Autodesk Inventor part; units mm, degrees
ref_plane "YZ Plane" through (0, 0, 0) normal (1, 0, 0) x (0, 1, 0)
ref_plane "XZ Plane" through (0, 0, 0) normal (0, 1, 0) x (-1, 0, 0)
ref_plane "XY Plane" through (0, 0, 0) normal (0, 0, 1) x (1, 0, 0)
sketch "Sketch1" plane through (0, 0, 0) normal (0, 0, 1) x (1, 0, 0)
  line L0 (0, 65.5357) -> (0, 44) construction
  line L1 (0, 0) -> (50, 0)
  line L2 (50, 0) -> (50, 5)
  line L3 (50, 5) -> (25, 5)
  line L4 (25, 5) -> (25, 68)
  line L5 (25, 68) -> (14, 68)
  line L6 (14, 68) -> (14, 58)
  arc A0 (0, 44) -> (14, 58) centre (0, 58) ccw
  circle A1 centre (17.75, 58) radius 2
  line L7 (0, 44) -> (0, 0)
  point P0 (0, 50)
  dimension "d0" = 5
  dimension "d1" = 50
  dimension "d2" = 25
  dimension "d4" = 14
  dimension "d5" = 4
  dimension "d6" = 17.75
  dimension "d7" = 10
  dimension "d22" = 50
  dimension "d23" = 6
extrude "Extrusion1" add sketch "Sketch1" along normal blind 18.2
mirror "Mirror1" about plane through (0, 0, 0) normal (1, 0, 0) of "Extrusion1"
sketch "Sketch2" plane through (50, 0, 0) normal (0, -1, 0) x (1, 0, 0)
  line L0 (-75, 0) -> (-75, 18.2)
  line L1 (-25, 0) -> (-25, 18.2)
  line L2 (-100, 0) -> (-100, 18.2)
  line L3 (0, 0) -> (0, 18.2)
  line L4 (0, 18.2) -> (-100, 18.2)
  line L5 (-100, 0) -> (0, 0)
  point P0 (-50, 0)
  point P1 (-93, 13.2)
  point P2 (-93, 5)
  point P3 (-7, 5)
  point P4 (-7, 13.2)
  dimension "d10" = 7
  dimension "d11" = 7
  dimension "d12" = 5
  dimension "d13" = 5
hole "Hole1" at (-43, 0, 13.2) at (-43, 0, 5) at (43, 0, 5) at (43, 0, 13.2) direction (0, 1, 0) diameter 4 end through all
fillet "Fillet1" radius 2 6 edges at (-50, 2.5, 18.2) (-50, 2.5, 0) (50, 2.5, 0) (50, 2.5, 18.2) (25, 68, 9.1) (-25, 68, 9.1)
properties part number "STEPPER MOTOR MOUNT"
The listing builds one solid part. Answer for the finished solid, in the listing's coordinates (mm). A direction names the side the tool comes from. Round coordinates to 2 decimals unless told otherwise and drop trailing zeros. Write each loop counter-clockwise with the first axis right and the second up, starting at its lowest first coordinate (ties: lowest second). Pieces come first, ordered by that corner, then holes. Notation, with made-up numbers: (23, -36) - (60, -36) arc R19 ccw to (60, -26) - close; hole circle Ø10 at (22.5, 66). An arc over 180 degrees is marked (long way). Use a Markdown table: item, result. Add a question column.
1. The part is cut by section C-C (y = 57). Write down the section's boundary in (x, z).
2. Flat-ended cylindrical pins translate along their axes: P1, Ø4.5, axis at x = -43, z = 5, coming from the +Y side; P2, Ø8, axis at y = 41, z = 11, coming from the +X side; P3, Ø5, axis at y = 63, z = 13, coming from the -X side. Find the tip coordinate at first contact, or state that the pin passes through.
3. A tool of negligible diameter and unlimited length cuts with its end or side. For faces 4 (the face through (-25, 36, 9)), 5 (the face through (38, 5, 9)), 6 (the face through (-1, 0, 9)), 7 (the face through (-14, 63, 9)), from which of +Z, -Z, +X, -X, +Y, -Y can it reach the whole face along a straight path? Write none if from no direction.
4. Consider line 1 (X direction, y = 1.8, z = 13.2); line 2 (Z direction, x = -43, y = 2.15); line 3 (Y direction, x = 17.75, z = 13.75). Determine where each line is inside the solid, lowest interval first.
5. The part is cut by section D-D (z = 8.25). Write down the section's boundary in (x, y).
6. The part is cut by section B-B (x = -17.75). Write down the section's boundary in (y, z).
7. The part is cut by section A-A (z = 13.2). Write down the section's boundary in (x, y).
8. For a pull along X with two mould halves and no side action, classify faces 1 (the face through (-18, 68, 9)), 2 (the face through (-50, 3, 9)), 3 (the face through (-17.49, 59.983, 8.973)) as +X half, -X half, draft (parallel to the pull), parting line (faces both ways), or undercut.
Reported:
| question | item | result |
|---|---|---|
| 1 | outline | (-25, 0) - (-19.48, 0) - (-19.48, 18.2) - (-25, 18.2) - close; (-16.02, 0) - (-13.96, 0) - (-13.96, 18.2) - (-16.02, 18.2) - close; (13.96, 0) - (16.02, 0) - (16.02, 18.2) - (13.96, 18.2) - close; (19.48, 0) - (25, 0) - (25, 18.2) - (19.48, 18.2) - close |
| 2 | P1 | y = 5 |
| 2 | P2 | x = 25 |
| 2 | P3 | x = -25 |
| 3 | face 4 | +Z, -Z, -X, +Y |
| 3 | face 5 | +Z, -Z, +X, +Y |
| 3 | face 6 | +Z, -Z, +X, -X, -Y |
| 3 | face 7 | +Z, -Z, +Y |
| 4 | line 1 | -50 to -45, -41 to 41, 45 to 50 |
| 4 | line 2 | 0 to 3, 7 to 11.2, 15.2 to 18.2 |
| 4 | line 3 | 0 to 56, 60 to 68 |
| 5 | outline | (-50, 0) - (50, 0) - (50, 5) - (25, 5) - (25, 66) arc R2 ccw to (23, 68) - (14, 68) - (14, 58) arc R14 cw to (-14, 58) - (-14, 68) - (-23, 68) arc R2 ccw to (-25, 66) - (-25, 5) - (-50, 5) - close; hole circle Ø4 at (-17.75, 58); hole circle Ø4 at (17.75, 58) |
| 6 | outline | (0, 0) - (56, 0) - (56, 18.2) - (0, 18.2) - close; (60, 0) - (68, 0) - (68, 18.2) - (60, 18.2) - close |
| 7 | outline | (-50, 0) - (-45, 0) - (-45, 5) - (-50, 5) - close; (-41, 0) - (41, 0) - (41, 5) - (25, 5) - (25, 66) arc R2 ccw to (23, 68) - (14, 68) - (14, 58) arc R14 cw to (-14, 58) - (-14, 68) - (-23, 68) arc R2 ccw to (-25, 66) - (-25, 5) - (-41, 5) - close; (45, 0) - (50, 0) - (50, 5) - (45, 5) - close; hole circle Ø4 at (-17.75, 58); hole circle Ø4 at (17.75, 58) |
| 8 | face 1 | draft |
| 8 | face 2 | -X half |
| 8 | face 3 | undercut |
